Could you check a few things on this model? Use its own coordinates, in mm. Face numbers are marked on the shaded views. Give positions to 0.01 mm unless a question says otherwise; leave off trailing zeros. Write each loop counter-clockwise with the first axis right and the second up, starting at its lowest first coordinate (ties: lowest second). Pieces come first, ordered by that corner, then holes. Notation, with made-up numbers: M 10.25,16 L 23.25,16 A29 ccw 23.25,54 Z; hole C 60,18 d5. An arc over 180 degrees is marked long. One line per item, written item: value.
```python
from build123d import *

# Parameters (mm, degrees)
F2_T = -1.27


with BuildPart() as f1:
    # F0 (on Front) → F1 (revolve)
    with BuildSketch(Plane.XZ):
        with BuildLine():
            ThreePointArc((-60.2397024632, 38.6090278625), (-58.6273197833, 25.5915278625), (-60.2397024632, 12.5740278625))
            Line((-60.2397024632, 12.5740278625), (-47.5397024632, 12.5740278625))
            Line((-47.5397024632, 12.5740278625), (-47.5397024632, 38.6090278625))
            Line((-47.5397024632, 38.6090278625), (-60.2397024632, 38.6090278625))
        make_face()
    revolve(axis=Axis((-28.491001968, 0, 25.3042703682), (0, 0, -1)))

    # F2
    f2_openings = [f1.faces().sort_by_distance(p)[0] for p in [
        (-9.442301, 0, 25.591528),
    ]]
    offset(amount=F2_T, openings=f2_openings)


solid = f1.part
```
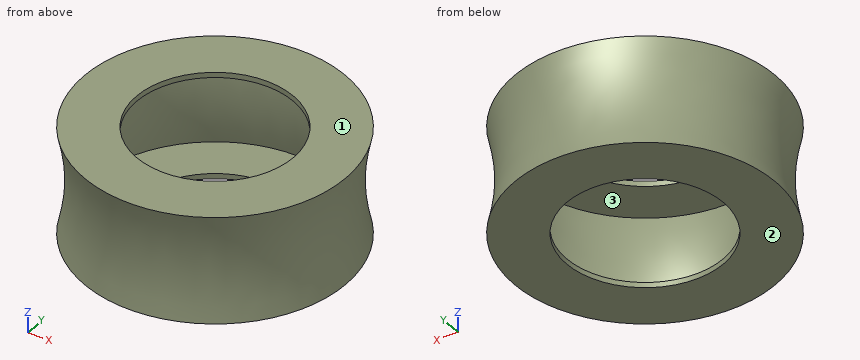
1) I'm going to push flat-ended pins straight in: pin 1 (8 mm diameter, centred on x = -16.5, z = 22.5, fed in from -Y); pin 2 (3 mm diameter, centred on x = -32, z = 29.5, fed in from +Y); pin 3 (2 mm diameter, centred on y = -17.5, z = 32.5, fed in from -X). Where does each tip first touch, or does it pass through?
Outcome:
pin 1: stops at y = -29.19
pin 2: stops at y = 30.27
pin 3: stops at x = -54.26
2) Please list where these lines run through material, in increasing order: L1, parallel to Z at x = -28.5, y = -24.5; L2, parallel to X at y = 4.5, z = 18.5; L3, parallel to X at y = -25.5, z = 34.5. Write a range as from..to.
Outcome:
L1: z = 12.57..13.84, 37.34..38.61
L2: x = -58.77..-57.47, 0.49..1.79
L3: x = -45.92..-43.52, -13.47..-11.07
3) If we section it at A-A, the plane y = 0: Write out the boundary of the cut face in (x, z), then the cut area to 3 significant figures.
Outcome:
outline: M -60.24,12.57 L -47.54,12.57 L -47.54,13.84 L -58.64,13.84 A54.62 ccw -58.64,37.34 L -47.54,37.34 L -47.54,38.61 L -60.24,38.61 A53.35 cw Z; M -9.44,12.57 L 3.26,12.57 A53.35 cw 3.26,38.61 L -9.44,38.61 L -9.44,37.34 L 1.65,37.34 A54.62 ccw 1.65,13.84 L -9.44,13.84 Z
area: 124 mm^2
4) If we section it at C-C, the plane z = 27.25: Write out the boundary of the cut face in (x, y), then the cut area to 3 significant figures.
Outcome:
outline: C -28.49,0 d60.32; hole C -28.49,0 d57.78
area: 236 mm^2
5) If we section it at B-B, the plane z = 34.75: Write out the boundary of the cut face in (x, y), then the cut area to 3 significant figures.
Outcome:
outline: C -28.49,0 d61.86; hole C -28.49,0 d59.28
area: 245 mm^2
6) We'd pull the mould along Z, two halves only. Please class the marked faces 1, 2 and 3: pulls with the +Z half, pulls with the -Z half, needs draft (parallel to the pull), parting line crosses it, or undercut.
Outcome:
face 1: pulls with the +Z half
face 2: pulls with the -Z half
face 3: undercut
